Here's the drawing with two shaded views (mm, measured from the low corner). I have some questions. A direction names the side the tool comes from. Round coordinates to 2 decimals unless told otherwise and drop trailing zeros. Order: outer loops, then holes, each group sorted by start corner. A loop starts at its lowest first (then second) coordinate and runs counter-clockwise, first axis right, second up.
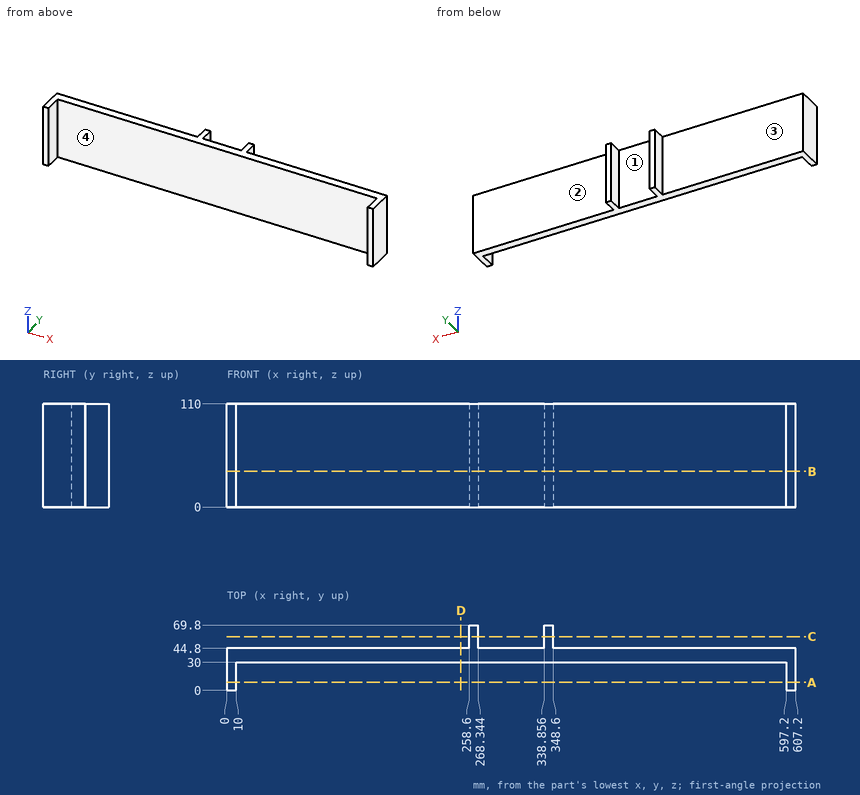
1. On a 3-axis mill with a long thin cutter (end or side, diameter ignored), from which of +Z, -Z, +X, -X, +Y, -Y can I reach the whole of each face in a straight line? I mean the marked faces 1 and 2. Say none if no direction works.
Evaluation:
face 1: +Z, -Z, +Y
face 2: +Z, -Z, +X, +Y
2. I'm going to push flat-ended pins straight in: P1, Ø10, axis at x = 345, z = 29.5, coming from the -Y side; P2, Ø1.5, axis at y = 40.5, z = 71, coming from the -X side; P3, Ø21, axis at x = 290.5, z = 42.5, coming from the +Y side; P4, Ø12.5, axis at y = 54.5, z = 56, coming from the -X side. Where does each tip first touch, or does it pass through?
Evaluation:
P1: stops at y = 30
P2: stops at x = 0
P3: stops at y = 44.8
P4: stops at x = 258.6
3. If we mould it in two halves opening along X, with no side actions, what happens to the marked faces 3 and 4? For each: released by +X, released by -X, zero draft, split by the parting line, or undercut.
Evaluation:
face 3: zero draft
face 4: undercut
4. If we section it at B-B, the plane z = 38: Write out the boundary of the cut face in (x, y) (1 decimal).
Evaluation:
outline: (0, 0) - (10, 0) - (10, 30) - (597.2, 30) - (597.2, 0) - (607.2, 0) - (607.2, 44.8) - (348.6, 44.8) - (348.6, 69.8) - (338.9, 69.8) - (338.9, 44.8) - (268.3, 44.8) - (268.3, 69.8) - (258.6, 69.8) - (258.6, 44.8) - (0, 44.8) - close
5. If we section it at D-D, the plane x = 250: Write out the boundary of the cut face in (y, z), and give its area (3 significant figures).
Evaluation:
outline: (30, 0) - (44.8, 0) - (44.8, 110) - (30, 110) - close
area: 1,630 mm2
6. If we section it at C-C, the plane y = 57.5: Write out the boundary of the cut face in (x, z) (1 decimal), and give its area (3 significant figures).
Evaluation:
outline: (258.6, 0) - (268.3, 0) - (268.3, 110) - (258.6, 110) - close; (338.9, 0) - (348.6, 0) - (348.6, 110) - (338.9, 110) - close
area: 2,140 mm2
7. I need wall thicknesses on probe 1 along X at (y, z) = (18, 20); probe 2 along X at (y, z) = (53, 51.5) (1 decimal); probe 3 along Y at (x, z) = (310.5, 88). Which ranges of each line are inside material? Lowest first, please.
Evaluation:
probe 1: x = 0 to 10, 597.2 to 607.2
probe 2: x = 258.6 to 268.3, 338.9 to 348.6
probe 3: y = 30 to 44.8
8. If we section it at A-A, the plane y = 8.5: Write out the boundary of the cut face in (x, z).
Evaluation:
outline: (0, 0) - (10, 0) - (10, 110) - (0, 110) - close; (597.2, 0) - (607.2, 0) - (607.2, 110) - (597.2, 110) - close
